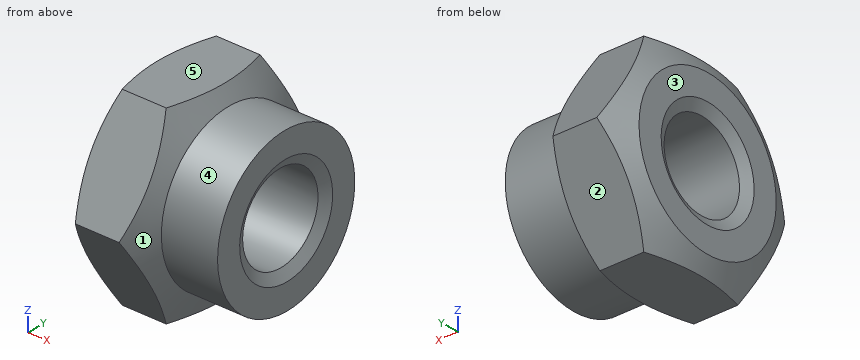
Autodesk Inventor part; units mm, degrees
ref_plane "Work Plane1" through (11.804, 0, 0) normal (0, 0, 1) x (-1, 0, 0)
ref_plane "YZ Plane" through (0, 0, 0) normal (1, 0, 0) x (0, 1, 0)
ref_plane "XZ Plane" through (0, 0, 0) normal (0, 1, 0) x (-1, 0, 0)
sketch "Skizze1" plane through (0, 0, 0) normal (1, 0, 0) x (0, 1, 0)
  line L0 (2.0207, -3.5) -> (-2.0207, -3.5)
  line L1 (-2.0207, -3.5) -> (-4.0415, 0)
  line L2 (-4.0415, 0) -> (-2.0207, 3.5)
  line L3 (-2.0207, 3.5) -> (2.0207, 3.5)
  line L4 (2.0207, 3.5) -> (4.0415, 0)
  line L5 (4.0415, 0) -> (2.0207, -3.5)
  point P0 (0, 0)
  point P1 (0, 0)
  dimension "d0" = 8.0829
extrude "Körper" add sketch "Skizze1" along normal blind 2.9
sketch "Skizze2" plane through (2.9, 0, 0) normal (1, 0, 0) x (0, 0, -1)
  circle A0 centre (0, 0) radius 2.95
  dimension "d7" = 5.9
extrude "Ring" add sketch "Skizze2" along normal blind 2.1
sketch "Skizze3" plane through (0, 0, 0) normal (0, 0, 1) x (1, 0, 0)
  line L0 (0, 2.0207) -> (0, 4.0415)
  line L1 (0, 4.0415) -> (2.9, 4.0415)
  line L2 (2.9, 2.0207) -> (2.9, 4.0415)
  line L3 (-0.58, 0) -> (3.48, 0)
  line L4 (0, 2.95) -> (0.6302, 4.0415)
  line L5 (2.2698, 4.0415) -> (2.9, 2.95)
  dimension "d3" = 30
  dimension "d4" = 30
  dimension "d5" = 5.9
  dimension "d6" = 5.9
revolve "Fase1" cut sketch "Skizze3" angle 360 about axis through (-10, 0, 0) along (1, 0, 0)
sketch "Skizze4" plane through (0, 0, 0) normal (-1, 0, 0) x (0, 0, 1)
  line L0 (0, -5.658) -> (0, 5.658)
  line L1 (-4.9, 0) -> (4.9, 0)
  point P0 (0, 0)
hole "Gewinde" at (0, 0, 0) direction (1, 0, 0) diameter 3.242 end through all
chamfer "Fase2" distance 0.3789 angle 30 1 edges at (0, 0, -1.621) measured on face at (0, 2.4745, -0.3005)
chamfer "Fase3" distance 0.3789 angle 30 1 edges at (5, 0, -1.621) measured on face at (5, -0.3646, -2.4627)
ref_plane "Work Plane1" through (11.804, 0, 0) normal (0, 0, 1) x (-1, 0, 0)
equation "\"d0\" = 1.1547 * SW"
equation "\"d1\" = KOH1"
equation "\"d7\" = SD2"
equation "\"d8\" = KOH - KOH1"
equation "\"d3\" = ANG1"
equation "\"d4\" = ANG2"
equation "\"d5\" = SW0"
equation "\"d6\" = SW01"
equation "\"d10\" = -0.5 * GD1 + 0.5 * NND"
equation "\"d46\" = -0.5 * GD1 + 0.5 * NND"
equation "\"d12\" = -0.5 * GD1 + 0.5 * NND"
equation "\"d47\" = -0.5 * GD1 + 0.5 * NND"
equation "\"ANG1\" = 30deg"
equation "\"ANG2\" = 30deg"
equation "\"NND\" = 4"
equation "\"KOH1\" = 2.9"
equation "\"KOH\" = 5"
equation "\"SW\" = 7"
equation "\"SW0\" = 5.9"
equation "\"SW01\" = SW0"
equation "\"SD2\" = SW0"
equation "\"GUL\" = 0.541266 * PTC"
equation "\"THREADDIA\" = 4"
equation "\"TOA\" = 30deg"
equation "\"PTC\" = 0.7"
equation "\"GAL\" = 0.541266 * PTC"
equation "\"E0\" = 1.155 * SW"
properties part number "DIN 985 - M4" material "Stahl, weich"
Verification items for the finished model (mm, model axes). Face numbers are marked on the shaded views. A direction names the side the tool comes from. Round coordinates to 2 decimals unless told otherwise and drop trailing zeros. Loops run counter-clockwise (first coordinate to the right, second up) from the corner with the lowest first, then second, coordinate; pieces in that order, holes last. Notation, with made-up numbers: (32.25, 65.25) - (54.25, 65.25) arc R9 ccw to (54.25, 69.25) - close; hole circle Ø1 at (-24.75, 69). An arc over 180 degrees is marked (long way). Use a Markdown table: item, result. Add a question column.
1. Section check B-B, the plane y = 0. Record the boundary of the cut face in (x, z).
2. Access from +Z, -Z, +X, -X, +Y, -Y to the whole of each face (thin tool, end or side, straight path). Record for the marked faces 4 and 5.
3. Release check for a two-part mould opening along X. For the marked faces 1, 2 and 3 record: released by +X, released by -X, zero draft, split by the parting line, or undercut.
4. Section check C-C, the plane x = 3.05. Record the boundary of the cut face in (y, z).
5. Thickness scan on probe 1 along Z at (x, y) = (1.75, 0); probe 2 along Y at (x, z) = (2.2, -1.25); probe 3 along Y at (x, z) = (2.75, 0). Record the ranges inside material, lowest first. Write a range as [from, to].
6. Gauge pin test, flat ends, axial feed: pin 1 (1.5 mm diameter, centred on x = 4, z = 2.5, fed in from -Y); pin 2 (1 mm diameter, centred on x = 0.5, z = 1.5, fed in from +Y); pin 3 (3 mm diameter, centred on x = 2, z = -2, fed in from -Y). Record the tip position at first contact, or that the pin passes through.
7. Section check A-A, the plane x = 1.25. Record the boundary of the cut face in (y, z), plus the area to 3 significant figures.
Checks:
| question | item | result |
|---|---|---|
| 1 | outline | (0, -2.95) - (0.32, -3.5) - (2.58, -3.5) - (2.9, -2.95) - (5, -2.95) - (5, -2) - (4.78, -1.62) - (0.22, -1.62) - (0, -2) - close; (0, 2) - (0.22, 1.62) - (4.78, 1.62) - (5, 2) - (5, 2.95) - (2.9, 2.95) - (2.58, 3.5) - (0.32, 3.5) - (0, 2.95) - close |
| 2 | face 4 | +X |
| 2 | face 5 | +Z, +X, -X, +Y, -Y |
| 3 | face 1 | released by +X |
| 3 | face 2 | zero draft |
| 3 | face 3 | released by -X |
| 4 | outline | circle Ø5.9 at (0, 0); hole circle Ø3.24 at (0, 0) |
| 5 | probe 1 | z = [-3.5, -1.62], [1.62, 3.5] |
| 5 | probe 2 | y = [-3.32, -1.03], [1.03, 3.32] |
| 5 | probe 3 | y = [-3.21, -1.62], [1.62, 3.21] |
| 6 | pin 1 | stops at y = -2.37 |
| 6 | pin 2 | stops at y = 3.46 |
| 6 | pin 3 | stops at y = -3.75 |
| 7 | outline | (-4.04, 0) - (-2.02, -3.5) - (2.02, -3.5) - (4.04, 0) - (2.02, 3.5) - (-2.02, 3.5) - close; hole circle Ø3.24 at (0, 0) |
| 7 | area | 34.2 mm^2 |
